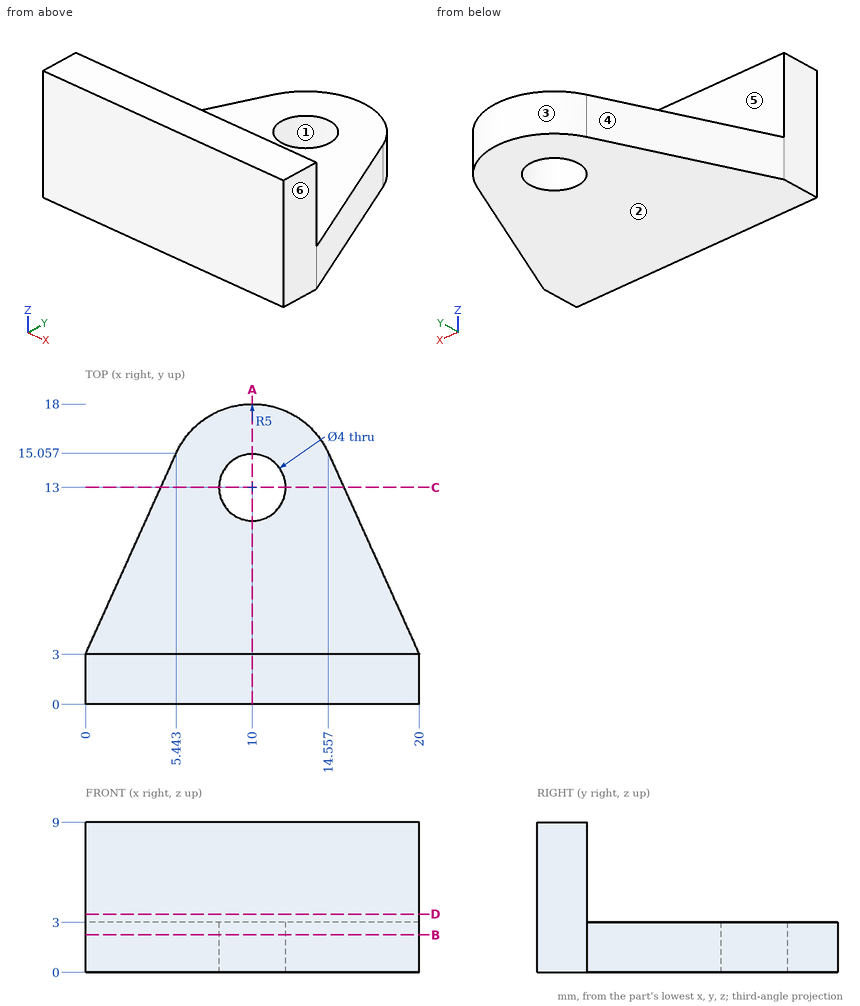
Geometry check sheet. Reference: drawing and pictorial views, mm from the part's lowest x, y, z. A direction names the side the tool comes from. Coordinates: 2 decimals unless noted, no trailing zeros. Write each loop counter-clockwise with the first axis right and the second up, starting at its lowest first coordinate (ties: lowest second). Pieces come first, ordered by that corner, then holes.
Item 1: Cross-section at D-D on z = 3.5. Record the boundary of the cut face in (x, y), then the cut area to 3 significant figures.
Numbers:
outline: (0, 0) - (20, 0) - (20, 3) - (0, 3) - close
area: 60.0 mm2
Item 2: Cross-section at A-A on x = 10. Record the boundary of the cut face in (y, z).
Numbers:
outline: (0, 0) - (11, 0) - (11, 3) - (3, 3) - (3, 9) - (0, 9) - close; (15, 0) - (18, 0) - (18, 3) - (15, 3) - close
Item 3: Cross-section at C-C on y = 13. Record the boundary of the cut face in (x, z).
Numbers:
outline: (4.51, 0) - (8, 0) - (8, 3) - (4.51, 3) - close; (12, 0) - (15.49, 0) - (15.49, 3) - (12, 3) - close
Item 4: Access from +Z, -Z, +X, -X, +Y, -Y to the whole of each face (thin tool, end or side, straight path). Record for the marked faces 5 and 6.
Numbers:
face 5: +Z, +X, -X, +Y
face 6: +Z, -Z, +X, +Y, -Y
Item 5: Scan lines: probe 1 along Y at (x, z) = (10, 1.9); probe 2 along Z at (x, y) = (4.5, 4). Record each from-to range of solid material in increasing order.
Numbers:
probe 1: y = 0 to 11, 15 to 18
probe 2: z = 0 to 3
Item 6: Mould release check, pull along X, two halves, no side actions. Record for the marked faces 1, 2, 3 and 4: released by +X, released by -X, zero draft, split by the parting line, or undercut.
Numbers:
face 1: undercut
face 2: zero draft
face 3: split by the parting line
face 4: released by -X
Item 7: Depth check by flat-ended pin: pin 1 Ø3 at (x, y) = (14, 15) entering from +Z; pin 2 Ø3.5 at (x, y) = (10, 13) entering from -Z. Enter the tip coordinate at first touch or a pass-through.
Numbers:
pin 1: stops at z = 3
pin 2: passes through
Item 8: Cross-section at B-B on z = 2.25. Record the boundary of the cut face in (x, y), then the cut area to 3 significant figures.
Numbers:
outline: (0, 0) - (20, 0) - (20, 3) - (14.56, 15.06) arc R5 ccw to (5.44, 15.06) - (0, 3) - close; hole circle Ø4 at (10, 13)
area: 242 mm2
